CAD build for the part. Positions are in the model's coordinates, mm. A direction names the side the tool comes from. Coordinates: 2 decimals unless noted, no trailing zeros. Loops run counter-clockwise (first coordinate to the right, second up) from the corner with the lowest first, then second, coordinate; pieces in that order, holes last. Notation, with made-up numbers: M 58,51.25 L 113,51.25 A8 ccw 113,55.25 Z; hole C 77,-30.5 d4. An arc over 180 degrees is marked long. Answer as a JSON object with one key per item and string values. Group by question number.
```python
from build123d import *

# Parameters (mm, degrees)
SKETCH1_R             = 3.5
SKETCH1_R_2           = 1.55
BOSS_EXTRUDE1_DEPTH   = 3.5
BOSS_EXTRUDE1_2_DEPTH = 3.5
BOSS_EXTRUDE1_3_DEPTH = 3.5
BOSS_EXTRUDE1_4_DEPTH = 3.5
BOSS_EXTRUDE2_DEPTH   = 0.2


with BuildPart() as part:
    # Sketch1 → Boss-Extrude1 (new body)
    with BuildSketch(Plane.XY):
        Circle(SKETCH1_R)
        Circle(SKETCH1_R_2, mode=Mode.SUBTRACT)
    extrude(amount=BOSS_EXTRUDE1_DEPTH)



with BuildPart() as body_2:
    # Sketch1 → Boss-Extrude1 2 (new body)
    with BuildSketch(Plane.XY):
        with Locations((10, 0)):
            Circle(SKETCH1_R)
        with Locations((10, 0)):
            Circle(SKETCH1_R_2, mode=Mode.SUBTRACT)
    extrude(amount=BOSS_EXTRUDE1_2_DEPTH)


with BuildPart() as body_3:
    # Sketch1 → Boss-Extrude1 3 (new body)
    with BuildSketch(Plane.XY):
        with Locations((10, 10)):
            Circle(SKETCH1_R)
        with Locations((10, 10)):
            Circle(SKETCH1_R_2, mode=Mode.SUBTRACT)
    extrude(amount=BOSS_EXTRUDE1_3_DEPTH)


with BuildPart() as body_4:
    # Sketch1 → Boss-Extrude1 4 (new body)
    with BuildSketch(Plane.XY):
        with Locations((0, 10)):
            Circle(SKETCH1_R)
        with Locations((0, 10)):
            Circle(SKETCH1_R_2, mode=Mode.SUBTRACT)
    extrude(amount=BOSS_EXTRUDE1_4_DEPTH)


with BuildPart() as part_1:
    add(part.part)

    add(body_2.part)  # Boss-Extrude2 merges body 2

    add(body_3.part)  # Boss-Extrude2 merges body 3

    add(body_4.part)  # Boss-Extrude2 merges body 4
    # Sketch2 → Boss-Extrude2 (add)
    with BuildSketch(Plane.XY):
        with BuildLine():
            Line((-3.5, 10), (-3.5, 0))
            ThreePointArc((-3.5, 0), (-2.474873734, -2.474873734), (0, -3.5))
            Line((0, -3.5), (10, -3.5))
            ThreePointArc((10, -3.5), (12.474873734, -2.474873734), (13.5, 0))
            Line((13.5, 0), (13.5, 10))
            ThreePointArc((13.5, 10), (12.474873734, 12.474873734), (10, 13.5))
            Line((10, 13.5), (0, 13.5))
            ThreePointArc((0, 13.5), (-2.474873734, 12.474873734), (-3.5, 10))
        make_face()
    extrude(amount=BOSS_EXTRUDE2_DEPTH)


solid = part_1.part
```
Item 1: Drill centre lines: L1, parallel to X at y = 10, z = 2.25; L2, parallel to Y at x = 0.75, z = 2.35. Where is each one in solid material? Low to high. Write a range as from..to.
Item 2: Slice it at C-C, the plane x = 4.5. Write the cut outline in (y, z), then the cut area to 3 significant figures.
Item 3: Pin check, flat tips, straight feed: pin 1 (0.9 mm diameter, centred on x = 0, y = 10, fed in from +Z); pin 2 (1.6 mm diameter, centred on x = -0.5, y = -1, fed in from +Z). Stop position of each tip, or through.
Item 4: Pull direction Y, two halves, no side cores. Call faces 3 (the flat face through (1, -2, 3.5)), 4 (the cylindrical face through (-2.58, 12.365, 1.726)): released by +Y, released by -Y, zero draft, split by the parting line, or undercut.
Item 5: Tool access for faces 1 (the flat face through (0, 10, 0.2)), 2 (the flat face through (12, -1, 3.5)): list every direction of +Z, -Z, +X, -X, +Y, -Y with a clear straight run to the whole face (end or side of a thin tool).
Item 6: Slice it at A-A, the plane z = 2.25. Write the cut outline in (x, y), then the cut area to 3 significant figures.
Item 7: Slice it at B-B, the plane y = 1.75. Write the cut outline in (x, z), then the cut area to 3 significant figures.
Computed:
{
 "1": {"L1": "-3.5..-1.55, 1.55..3.5, 6.5..8.45, 11.55..13.5", "L2": "-3.42..-1.36, 1.36..3.42, 6.58..8.64, 11.36..13.42"},
 "2": {"outline": "M -3.5,0 L 13.5,0 L 13.5,0.2 L -3.5,0.2 Z", "area": "3.40 mm2"},
 "3": {"pin 1": "z = 0.2", "pin 2": "z = 3.5"},
 "4": {"face 3": "zero draft", "face 4": "undercut"},
 "5": {"face 1": "+Z", "face 2": "+Z, +X, -X, +Y, -Y"},
 "6": {"outline": "C 0,0 d7; C 0,10 d7; C 10,0 d7; C 10,10 d7; hole C 0,0 d3.1; hole C 0,10 d3.1; hole C 10,0 d3.1; hole C 10,10 d3.1", "area": "124 mm2"},
 "7": {"outline": "M -3.5,0 L 13.5,0 L 13.5,0.2 L 13.03,0.2 L 13.03,3.5 L 6.97,3.5 L 6.97,0.2 L 3.03,0.2 L 3.03,3.5 L -3.03,3.5 L -3.03,0.2 L -3.5,0.2 Z", "area": "43.4 mm2"}
}
